```python
from build123d import *

# Parameters (mm, degrees)
F0_W     = 30
F0_H     = 13
F1_DEPTH = 157
F2_W     = 30
F2_H     = 26
F3_DEPTH = 8
F4_W     = 30
F4_H     = 6.5
F5_DEPTH = 13
F6_W     = 30
F6_H     = 26
F7_DEPTH = 8


with BuildPart() as f1:
    # F0 (on Top) → F1 (new body)
    with BuildSketch(Plane.XY):
        Rectangle(F0_W, F0_H)
    extrude(amount=F1_DEPTH)

    # F2 (on face) → F3 (join)
    with BuildSketch(Plane(origin=(0, 0, 0), x_dir=(1, 0, 0), z_dir=(0, 0, -1))):
        Rectangle(F2_W, F2_H)
    extrude(amount=F3_DEPTH)

    # F4 (on face) → F5 (join)
    with BuildSketch(Plane(origin=(0, 0, -8), x_dir=(1, 0, 0), z_dir=(0, 0, -1))):
        with Locations((0, -9.75)):
            Rectangle(F4_W, F4_H)
        with Locations((0, 9.75)):
            Rectangle(F4_W, F4_H)
    extrude(amount=F5_DEPTH)

    # F6 (on face) → F7 (join)
    with BuildSketch(Plane(origin=(0, 0, -21), x_dir=(1, 0, 0), z_dir=(0, 0, -1))):
        Rectangle(F6_W, F6_H)
    extrude(amount=F7_DEPTH)


solid = f1.part
```
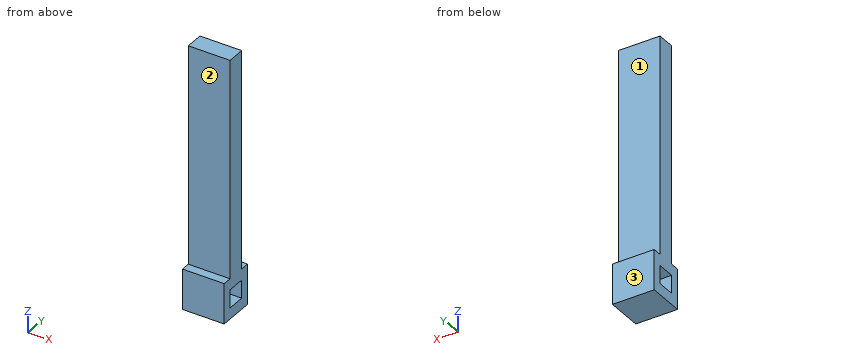
Build history of the part. All positions in model axes, mm. Face numbers are marked on the shaded views. A direction names the side the tool comes from. Give positions to 0.01 mm unless a question says otherwise; leave off trailing zeros. Loops run counter-clockwise (first coordinate to the right, second up) from the corner with the lowest first, then second, coordinate; pieces in that order, holes last. Notation, with made-up numbers: (89.5, 43) -> (140.5, 43) arc R12 cw to (140.5, 50) -> close; hole circle Ø1 at (-5.75, -2.75). An arc over 180 degrees is marked (long way). One line per question, with ' | ' between items. Start each with the question number.
1) Cut at B-B (x = 10.75). Give the cut face in (y, z), plus the area to 3 significant figures.
2) Cut at A-A (y = -4.25). Give the cut face in (x, z), plus the area to 3 significant figures.
3) Cut at D-D (z = 10). Give the cut face in (x, y).
4) Probe L1, parallel to Z at x = 8.5, y = -4; L2, parallel to Y at x = 8.5, z = -18.5; L3, parallel to Y at x = 0.75, z = 81. List the from-to ranges inside material, lowest first.
5) Cut at C-C (z = -15.5). Give the cut face in (x, y), plus the area to 3 significant figures.
6) 3-axis set-ups, long thin cutter, end or side, ignore diameter. For the marked faces 1, 2 and 3: which of +Z, -Z, +X, -X, +Y, -Y reach the whole face in a straight line?
7) Pin check, flat tips, straight feed: pin 1 (12 mm diameter, centred on x = 5.5, z = 83.5, fed in from +Y); pin 2 (5 mm diameter, centred on x = -4, z = 100, fed in from -Y); pin 3 (2 mm diameter, centred on x = -11, y = 8, fed in from +Z). Stop position of each tip, or through.
Return value:
1) outline: (-13, -29) -> (13, -29) -> (13, 0) -> (6.5, 0) -> (6.5, 157) -> (-6.5, 157) -> (-6.5, 0) -> (-13, 0) -> close; hole (-6.5, -21) -> (6.5, -21) -> (6.5, -8) -> (-6.5, -8) -> close | area: 2,630 mm^2
2) outline: (-15, -29) -> (15, -29) -> (15, -21) -> (-15, -21) -> close; (-15, -8) -> (15, -8) -> (15, 157) -> (-15, 157) -> close | area: 5,190 mm^2
3) outline: (-15, -6.5) -> (15, -6.5) -> (15, 6.5) -> (-15, 6.5) -> close
4) L1: -29 to -21, -8 to 157 | L2: -13 to -6.5, 6.5 to 13 | L3: -6.5 to 6.5
5) outline: (-15, -13) -> (15, -13) -> (15, -6.5) -> (-15, -6.5) -> close; (-15, 6.5) -> (15, 6.5) -> (15, 13) -> (-15, 13) -> close | area: 390 mm^2
6) face 1: +Z, +X, -X, +Y | face 2: +Z, +X, -X, -Y | face 3: +Z, -Z, +X, -X, +Y
7) pin 1: y = 6.5 | pin 2: y = -6.5 | pin 3: z = 0
